Check sheet for the modelled part. Datum: model origin and axes. Units: mm. A direction names the side the tool comes from. Coordinates: 2 decimals unless noted, no trailing zeros.
```python
from build123d import *

# Parameters (mm, degrees)
SKETCH1_W           = 80
SKETCH1_H           = 80
BOSS_EXTRUDE1_DEPTH = 5
FILLET1_R           = 2.5
BOSS_EXTRUDE5_DEPTH = 2
SKETCH12_R          = 33.6
SKETCH12_R_2        = 31.6
BOSS_EXTRUDE8_DEPTH = 3
SKETCH13_R          = 22
SKETCH13_R_2        = 20.5
BOSS_EXTRUDE9_DEPTH = 3
FILLET2_R           = 1.5
FILLET3_R           = 5


with BuildPart() as part:
    # Sketch1 → Boss-Extrude1 (new body)
    with BuildSketch(Plane.XY):
        Rectangle(SKETCH1_W, SKETCH1_H)
    extrude(amount=BOSS_EXTRUDE1_DEPTH)

    # Fillet1
    fillet1_edges = [part.edges().sort_by_distance(p)[0] for p in [
        (40, -40, 2.5),
        (-40, -40, 2.5),
        (-40, 40, 2.5),
        (40, 40, 2.5),
    ]]
    fillet(fillet1_edges, radius=FILLET1_R)

    # Sketch5 → Boss-Extrude5 (add)
    with BuildSketch(Plane.XY.offset(5)):
        with BuildLine():
            ThreePointArc((7.5, 28.013389656), (3.782307496, 28.752289474), (0, 29))
            ThreePointArc((0, 29), (-3.782307496, 28.752289474), (-7.5, 28.013389656))
            Line((-7.5, 28.013389656), (-7.5, 26.97684192))
            ThreePointArc((-7.5, 26.97684192), (0, 28), (7.5, 26.97684192))
            Line((7.5, 26.97684192), (7.5, 28.013389656))
        make_face()
        with BuildLine():
            ThreePointArc((7.5, -26.97684192), (0, -28), (-7.5, -26.97684192))
            Line((-7.5, -26.97684192), (-7.5, -28.013389656))
            ThreePointArc((-7.5, -28.013389656), (-3.782307496, -28.752289474), (0, -29))
            ThreePointArc((0, -29), (3.782307496, -28.752289474), (7.5, -28.013389656))
            Line((7.5, -28.013389656), (7.5, -26.97684192))
        make_face()
        with BuildLine():
            Line((-26.97684192, 7.5), (-28.013389656, 7.5))
            ThreePointArc((-28.013389656, 7.5), (-28.752289466, 3.782307556), (-29, 1.22e-07))
            ThreePointArc((-29, 1.22e-07), (-28.752289482, -3.782307436), (-28.013389656, -7.5))
            Line((-28.013389656, -7.5), (-26.97684192, -7.5))
            ThreePointArc((-26.97684192, -7.5), (-28, 0), (-26.97684192, 7.5))
        make_face()
        with BuildLine():
            ThreePointArc((29, 0), (28.752289474, 3.782307496), (28.013389656, 7.5))
            Line((28.013389656, 7.5), (26.97684192, 7.5))
            ThreePointArc((26.97684192, 7.5), (27.743031321, 3.78473422), (28, 0))
            ThreePointArc((28, 0), (27.743031321, -3.78473422), (26.97684192, -7.5))
            Line((26.97684192, -7.5), (28.013389656, -7.5))
            ThreePointArc((28.013389656, -7.5), (28.752289474, -3.782307496), (29, 0))
        make_face()
    extrude(amount=BOSS_EXTRUDE5_DEPTH)

    # Sketch12 → Boss-Extrude8 (add)
    with BuildSketch(Plane.XY.offset(5)):
        Circle(SKETCH12_R)
        Circle(SKETCH12_R_2, mode=Mode.SUBTRACT)
    extrude(amount=BOSS_EXTRUDE8_DEPTH)

    # Sketch13 → Boss-Extrude9 (add)
    with BuildSketch(Plane.XY.offset(5)):
        Circle(SKETCH13_R)
        Circle(SKETCH13_R_2, mode=Mode.SUBTRACT)
    extrude(amount=BOSS_EXTRUDE9_DEPTH)

    # Fillet2
    fillet2_edges = [part.edges().sort_by_distance(p)[0] for p in [
        (0, 29, 5),
        (29, 0, 5),
        (-29, 0, 5),
        (0, -29, 5),
    ]]
    fillet(fillet2_edges, radius=FILLET2_R)

    # Fillet3
    # the kernel refuses this fillet: 5 mm, written as the material it adds along each edge
    with BuildSketch(Plane(origin=(0, 0, 5), x_dir=(1, 0, 0), z_dir=(0, -1, 0))) as fillet3_piece_1:
        with BuildLine():
            CenterArc((38.182575695, 5), FILLET3_R, 203.578178478, 66.421821522)
            Line((38.182575695, 0), (38.182575695, -0.1))
            Line((38.182575695, -0.1), (33.6, -0.1))
            Line((33.6, -0.1), (33.5, 0))
            ThreePointArc((33.5, 0), (33.5, 1.5), (33.508348486, 2.96))
            Line((33.508348486, 2.96), (33.6, 3))
        make_face()
    revolve(axis=Axis((0, 0, 5), (0, 0, 1)))
    with BuildSketch(Plane(origin=(0, 0, 5), x_dir=(1, 0, 0), z_dir=(0, -1, 0))) as fillet3_piece_2:
        with BuildLine():
            CenterArc((15.917424305, 5), FILLET3_R, 270, 66.421821522)
            Line((15.917424305, 0), (15.917424305, -0.1))
            Line((15.917424305, -0.1), (20.5, -0.1))
            Line((20.5, -0.1), (20.6, 0))
            ThreePointArc((20.6, 0), (20.6, 1.5), (20.591651514, 2.96))
            Line((20.591651514, 2.96), (20.5, 3))
        make_face()
    revolve(axis=Axis((0, 0, 5), (0, 0, 1)))


solid = part.part
```
1) Depth check by flat-ended pin: pin 1 (0.6 mm diameter, centred on x = -27.5, z = 6.5, fed in from +Y); pin 2 (16 mm diameter, centred on x = 1.5, y = 1, fed in from +Z); pin 3 (0.6 mm diameter, centred on x = 28, z = 6.5, fed in from +Y). Enter the tip coordinate at first touch or a pass-through.
Answer sheet:
pin 1: stops at y = 21.66
pin 2: stops at z = 5
pin 3: stops at y = 21.01
2) Set-up check for faces 4 (the cylindrical face through (-39.287, 39.248, 2.535)), 5 (the flat face through (-24, 30, 5)): record each of +Z, -Z, +X, -X, +Y, -Y from which the full face is reachable in a straight line by a thin tool's end or side.
Answer sheet:
face 4: +Z, -Z, -X, +Y
face 5: +Z
3) Mould release check, pull along Y, two halves, no side actions. Record for faces 1 (the flat face through (27.7, 7.5, 6)), 2 (the flat face through (-1, -40, 2)), 3 (the flat face through (15, -15, 8)): +Y half, -Y half, draft (parallel to the pull), parting line (faces both ways), or undercut.
Answer sheet:
face 1: undercut
face 2: -Y half
face 3: draft
4) Scan lines: line 1 (Y direction, x = -4, z = 7.5); line 2 (Y direction, x = 0, z = 6.8); line 3 (Y direction, x = 0, z = 7.15). Record each from-to range of solid material in increasing order.
Answer sheet:
line 1: y = -33.62 to -31.35, -21.63 to -19.85, 19.85 to 21.63, 31.35 to 33.62
line 2: y = -34.34 to -31.6, -29 to -28, -22 to -19.76, 19.76 to 22, 28 to 29, 31.6 to 34.34
line 3: y = -34.07 to -31.6, -22 to -20.03, 20.03 to 22, 31.6 to 34.07
